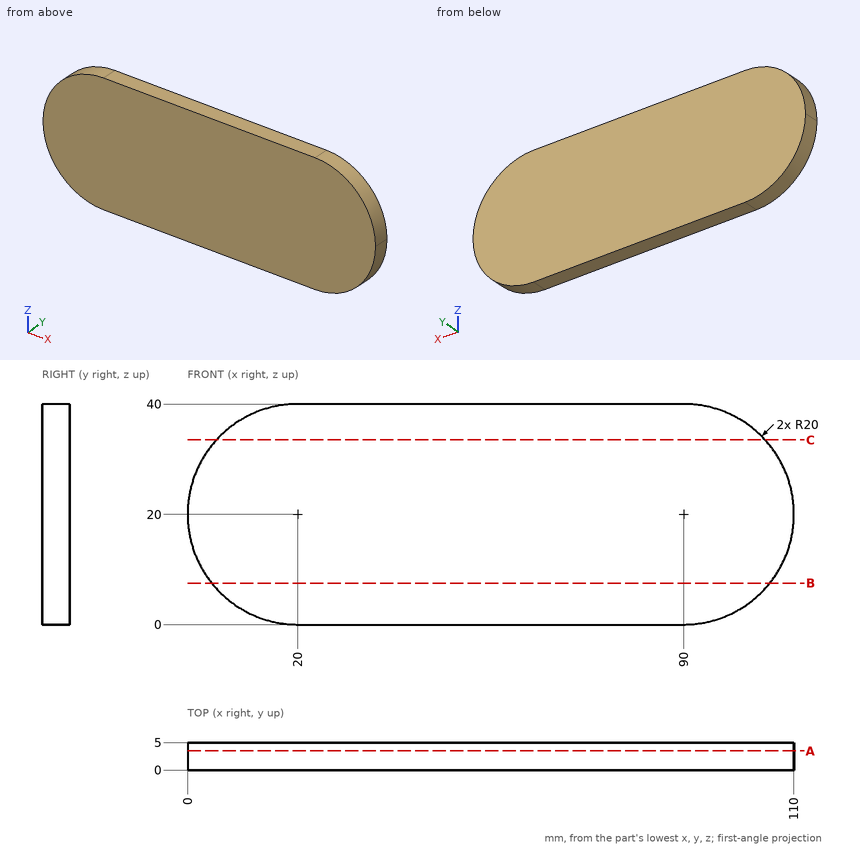
Can you work these out from the drawing? Everything is in mm from the part's minimum corner. Give positions to 0.01 mm unless a question says otherwise; leave off trailing zeros. Write each loop counter-clockwise with the first axis right and the second up, starting at its lowest first coordinate (ties: lowest second). Pieces come first, ordered by that corner, then holes. Notation, with made-up numbers: (22.25, 29) -> (29.25, 29) arc R18 ccw to (29.25, 52) -> close; hole circle Ø2 at (-6, -9.5). An arc over 180 degrees is marked (long way). Write each question's results on one line, items separated by ' | '.
Item 1: Suppose I cut it at C-C on z = 33.5. Write out the boundary of the cut face in (x, y), plus the area to 3 significant figures.
Output:
outline: (5.24, 0) -> (104.76, 0) -> (104.76, 5) -> (5.24, 5) -> close | area: 498 mm^2
Item 2: If I drill on L1, parallel to X at y = 1.9, z = 19.5; L2, parallel to X at y = 4.4, z = 9; L3, parallel to Z at x = 92, y = 4.6, over which ranges is the centre line in solid material (lowest first)?
Output:
L1: x = 0.01 to 109.99 | L2: x = 3.3 to 106.7 | L3: z = 0.1 to 39.9
Item 3: Suppose I cut it at B-B on z = 7.5. Write out the boundary of the cut face in (x, y), plus the area to 3 significant figures.
Output:
outline: (4.39, 0) -> (105.61, 0) -> (105.61, 5) -> (4.39, 5) -> close | area: 506 mm^2
Item 4: Suppose I cut it at A-A on y = 3.5. Write out the boundary of the cut face in (x, z), plus the area to 3 significant figures.
Output:
outline: (0, 20) arc R20 ccw to (20, 0) -> (90, 0) arc R20 ccw to (110, 20) arc R20 ccw to (90, 40) -> (20, 40) arc R20 ccw to start | area: 4,060 mm^2
